Autodesk Inventor part; units mm, degrees
ref_plane "YZ Plane" through (0, 0, 0) normal (1, 0, 0) x (0, 1, 0)
ref_plane "XZ Plane" through (0, 0, 0) normal (0, 1, 0) x (-1, 0, 0)
ref_plane "XY Plane" through (0, 0, 0) normal (0, 0, 1) x (1, 0, 0)
sketch "Sketch1" plane through (0, 0, 0) normal (0, 0, 1) x (1, 0, 0)
  arc A0 (1.5, 3.8) -> (0, 5.3) centre (0, 3.8) ccw
  line L0 (1.5, 3.8) -> (1.5, 1)
  line L1 (1.5, 1) -> (2, 1)
  line L2 (2, 1) -> (2, 0)
  line L3 (2, 0) -> (0, 0)
  line L4 (0, 0) -> (0, 5.3)
  point P0 (0, 0)
  dimension "d0" = 3
  dimension "d1" = 2
  dimension "d2" = 1
  dimension "d3" = 5.3
  dimension "d4" = 0
  dimension "d5" = 0
  dimension "d6" = 0
revolve "Revolution1" add sketch "Sketch1" angle 360 about axis through (0, 0, 0) along (0, 1, 0)
sketch "Sketch2" plane through (0, 0, 0) normal (0, 1, 0) x (-1, 0, 0)
  line L0 (-2.5, -4.5) -> (2.5, -4.5)
  line L1 (2.5, -4.5) -> (2.5, -1.5)
  line L2 (2.5, -1.5) -> (-2.5, -1.5)
  line L3 (-2.5, -1.5) -> (-2.5, -4.5)
  line L4 (-2.5, -4.5) -> (2.5, -1.5) construction
  line L5 (2.5, -4.5) -> (-2.5, -1.5) construction
  point P0 (0, 0)
  point P1 (0, -3)
  dimension "d8" = 1.5
  dimension "d9" = 5
  dimension "d10" = 3
  dimension "d12" = 2.5
extrude "Extrusion1" cut sketch "Sketch2" along normal blind 10
sketch "Sketch3" plane through (0, 0, 0) normal (0, -1, 0) x (1, 0, 0)
  arc A0 (1.3229, -1.5) -> (-1.3229, -1.5) centre (0, 0) ccw
  line L0 (-0.25, -1.52) -> (0.25, -1.52)
  line L1 (0.25, -1.52) -> (0.25, -1.02)
  line L2 (0.25, -1.02) -> (-0.25, -1.02)
  line L3 (-0.25, -1.02) -> (-0.25, -1.52)
  line L4 (-0.25, -1.52) -> (0.25, -1.02) construction
  line L5 (0.25, -1.52) -> (-0.25, -1.02) construction
  line L6 (-0.25, 1.02) -> (0.25, 1.02)
  line L7 (0.25, 1.02) -> (0.25, 1.52)
  line L8 (0.25, 1.52) -> (-0.25, 1.52)
  line L9 (-0.25, 1.52) -> (-0.25, 1.02)
  line L10 (-0.25, 1.02) -> (0.25, 1.52) construction
  line L11 (0.25, 1.02) -> (-0.25, 1.52) construction
  point P0 (0, -1.27)
  point P1 (0, 1.27)
  dimension "d15" = 0.5
  dimension "d16" = 0.5
  dimension "d17" = 0.5
  dimension "d18" = 0.5
  dimension "d19" = 2.54
  dimension "d20" = 1.27
extrude "Extrusion2" add sketch "Sketch3" along normal blind 3
properties part number "LED3mm"
The model under review builds one solid part; all positions refer to its coordinate system, in mm. A direction names the side the tool comes from. Coordinates: 2 decimals unless noted, no trailing zeros. Order: outer loops, then holes, each group sorted by start corner. A loop starts at its lowest first (then second) coordinate and runs counter-clockwise, first axis right, second up. Notation, with made-up numbers: (0, 78.5) -> (15, 78.5) arc R28 ccw to (15, 106.5) -> close; hole circle Ø5 at (-17, -30). An arc over 180 degrees is marked (long way). Answer in a Markdown table with one row per item. Add a question column.
Item 1: Clearance check with flat-ended pins moving along their axes: pin 1 (2 mm diameter, centred on x = 0, y = 2.5, fed in from -Z); pin 2 (0.6 mm diameter, centred on x = 0, y = -1, fed in from +Z). State where each tip first meets the part, or that it passes through.
Item 2: We need section B-B on y = 3. Write out the cut boundary in (x, z).
Item 3: We need section D-D on z = 1.4. Write out the cut boundary in (x, y), plus the area to 3 significant figures.
Item 4: We need section A-A on z = 0. Write out the cut boundary in (x, y).
Item 5: Machinability: for faces 1 (the cylindrical face through (0.07, 0.49, 2)), 2 (the flat face through (0, 1, 1.7)), which of the approach directions +Z, -Z, +X, -X, +Y, -Y give a long, thin tool a straight path to every point of the face, cutting with its end or side? Answer none if there is none.
Item 6: To check wall thickness, follow probe 1 along Z at (x, y) = (-0.2, -0.5); probe 2 along Z at (x, y) = (-0.85, 4.5); probe 3 along X at (y, z) = (-0.25, -1.1). State the ranges of each line that lie inside material, in increasing order.
Item 7: We need section C-C on x = 1.1. Write out the cut boundary in (y, z), plus the area to 3 significant figures.
Final values:
| question | item | result |
|---|---|---|
| 1 | pin 1 | stops at z = -1.5 |
| 1 | pin 2 | stops at z = 1.52 |
| 2 | outline | circle Ø3 at (0, 0) |
| 3 | outline | (-1.43, 0) -> (-0.25, 0) -> (-0.25, -3) -> (0.25, -3) -> (0.25, 0) -> (1.43, 0) -> (1.43, 1) -> (0.54, 1) -> (0.54, 3.8) arc R0.54 ccw to (-0.54, 3.8) -> (-0.54, 1) -> (-1.43, 1) -> close |
| 3 | area | 7.83 mm2 |
| 4 | outline | (-2, 0) -> (2, 0) -> (2, 1) -> (1.5, 1) -> (1.5, 3.8) arc R1.5 ccw to (-1.5, 3.8) -> (-1.5, 1) -> (-2, 1) -> close |
| 5 | face 1 | +Y, -Y |
| 5 | face 2 | +Y |
| 6 | probe 1 | z = -1.52 to -1.02, 1.02 to 1.52 |
| 6 | probe 2 | z = -1.02 to 1.02 |
| 6 | probe 3 | x = -0.25 to 0.25 |
| 7 | outline | (0, -1.5) -> (1, -1.5) -> (1, -1.02) -> (3.8, -1.02) arc R1.02 ccw to (3.8, 1.02) -> (1, 1.02) -> (1, 1.67) -> (0, 1.67) -> close |
| 7 | area | 10.5 mm2 |
